from build123d import *

# Parameters (mm, degrees)
SKETCH_1_R      = 5
EXTRUDE_1_DEPTH = 45


with BuildPart() as part:
    # ｽｹｯﾁ1 → ﾎﾞｽ - 押し出し1 (new body)
    with BuildSketch(Plane.XY):
        with Locations(Location((0, 0, 0), (0, 0, 180))):
            Circle(SKETCH_1_R)
    extrude(amount=EXTRUDE_1_DEPTH)

    # ｽｹｯﾁ3 → M4x0.7 ねじ穴1 (revolve, cut)
    with BuildSketch(Plane(origin=(0, 0, 45), x_dir=(0, -1, 0), z_dir=(1, 0, 0))):
        Polygon((0, 0), (0, 15.991420021), (1.65, 15), (1.65, 0), align=None)
    m4x0_7_1 = revolve(axis=Axis((0, 0, 51.35), (0, 0, -1)), mode=Mode.SUBTRACT)

    # ﾐﾗｰ1: M4x0.7 ねじ穴1 across plane
    add(m4x0_7_1.mirror(Plane.XY.offset(22.5)), mode=Mode.SUBTRACT)


solid = part.part
Verification items for the finished model (mm, model axes). A direction names the side the tool comes from. Give positions to 0.01 mm unless a question says otherwise; leave off trailing zeros. Loops run counter-clockwise (first coordinate to the right, second up) from the corner with the lowest first, then second, coordinate; pieces in that order, holes last. Notation, with made-up numbers: (31.25, -40) - (76.25, -40) arc R27 cw to (76.25, -22) - close; hole circle Ø8 at (88.5, 3). An arc over 180 degrees is marked (long way). Write each question's results on one line, items separated by ' | '.
1) Material ranges on L1, parallel to Y at x = 0, z = 11; L2, parallel to X at y = -1, z = 38; L3, parallel to Y at x = -3.25, z = 6.5, recorded low to high. Write a range as from..to.
Solution:
L1: -5..-1.65, 1.65..5 | L2: -4.9..-1.31, 1.31..4.9 | L3: -3.8..3.8
2) Sectioned sample at A-A on y = -3. Record the boundary of the cut face in (x, z), plus the area to 3 significant figures.
Solution:
outline: (-4, 0) - (4, 0) - (4, 45) - (-4, 45) - close | area: 360 mm2
3) Tool access check on faces 4 (the cylindrical face through (-1.115, 1.216, 7.395)), 5 (the flat face through (-2, 0, 45)), 6 (the cylindrical face through (-1.115, 1.216, 37.605)). Record the directions out of +Z, -Z, +X, -X, +Y, -Y that give a thin tool (end or side, any length) a straight path to the whole face; none if there is none.
Solution:
face 4: -Z | face 5: +Z, +X, -X, +Y, -Y | face 6: +Z
4) Depth check by flat-ended pin: P1, Ø1, axis at y = -2.5, z = 38, coming from the -X side; P2, Ø1, axis at x = 3, z = 7.5, coming from the +Y side; P3, Ø3, axis at x = 0, y = 0, coming from the +Z side. Enter the tip coordinate at first touch or a pass-through.
Solution:
P1: x = -4.58 | P2: y = 4.33 | P3: z = 29.91
5) Mould release check, pull along Y, two halves, no side actions. Record for faces 1 (the conical face through (0.1, -0.3, 29.2)), 2 (the cylindrical face through (5, 0, 22)), 3 (the flat face through (-2, 0, 0)): pulls with the +Y half, pulls with the -Y half, needs draft (parallel to the pull), parting line crosses it, or undercut.
Solution:
face 1: undercut | face 2: parting line crosses it | face 3: needs draft
